Job drawing, mm, ordinate dimensions from the low corner. One solid piece. A direction names the side the tool comes from. Give positions to 0.01 mm unless a question says otherwise; leave off trailing zeros. Loops run counter-clockwise (first coordinate to the right, second up) from the corner with the lowest first, then second, coordinate; pieces in that order, holes last. Notation, with made-up numbers: M 4,-19 L 36,-19 A20 cw 36,13 Z; hole C 79.5,-10 d6. An arc over 180 degrees is marked long. Answer in a Markdown table with one row per item.
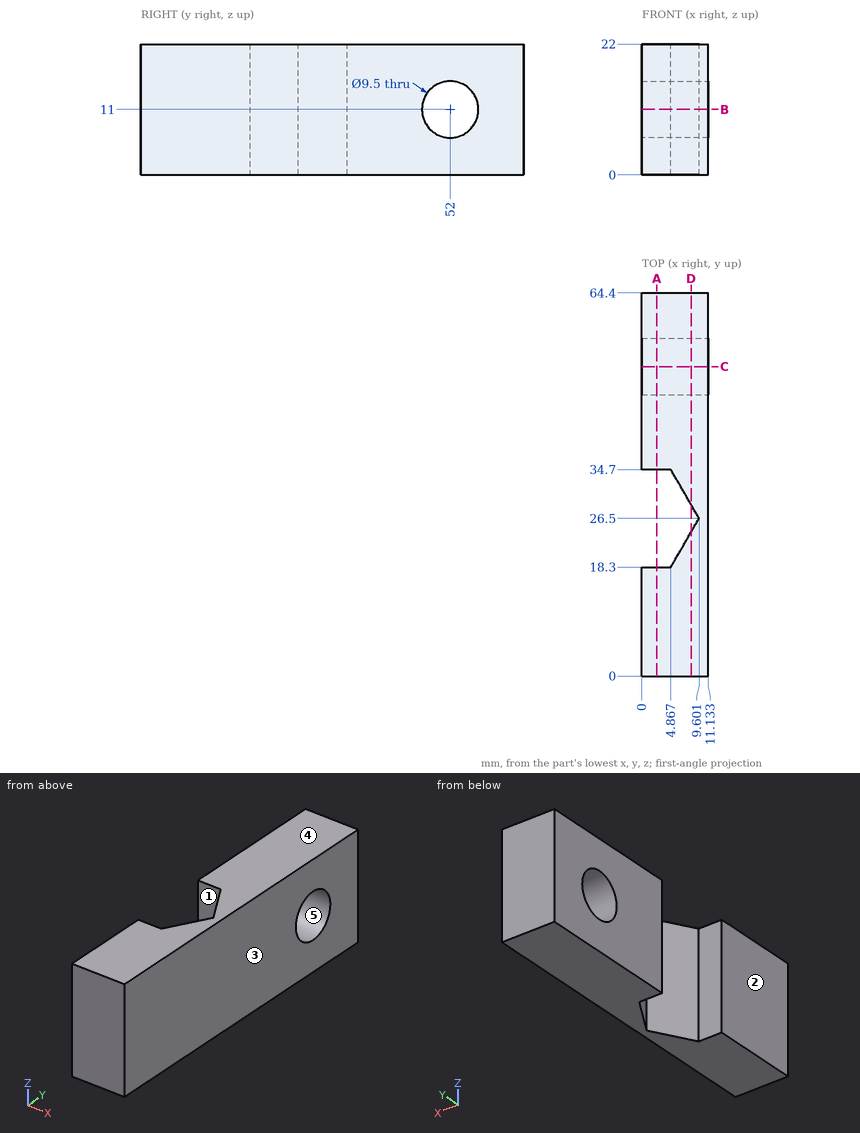
(1) Saw through at B-B (z = 11). Write the cut outline in (x, y).
Recorded:
| item | result |
|---|---|
| outline | M 0,0 L 11.13,0 L 11.13,47.25 L 0,47.25 L 0,34.7 L 4.87,34.7 L 9.6,26.5 L 4.87,18.3 L 0,18.3 Z; M 0,56.75 L 11.13,56.75 L 11.13,64.4 L 0,64.4 Z |
(2) Saw through at D-D (x = 8.25). Write the cut outline in (y, z).
Recorded:
| item | result |
|---|---|
| outline | M 0,0 L 24.16,0 L 24.16,22 L 0,22 Z; M 28.84,0 L 64.4,0 L 64.4,22 L 28.84,22 Z; hole C 52,11 d9.5 |
(3) Saw through at A-A (x = 2.5). Write the cut outline in (y, z), plus the area to 3 significant figures.
Recorded:
| item | result |
|---|---|
| outline | M 0,0 L 18.3,0 L 18.3,22 L 0,22 Z; M 34.7,0 L 64.4,0 L 64.4,22 L 34.7,22 Z; hole C 52,11 d9.5 |
| area | 985 mm^2 |
(4) Drill centre lines: line 1 along Y through (x, z) = (3, 11); line 2 along Y through (x, z) = (2.5, 4.25); line 3 along Y through (x, z) = (3.5, 9.5). Where is each one in solid material? Low to high.
Recorded:
| item | result |
|---|---|
| line 1 | y = 0 to 18.3, 34.7 to 47.25, 56.75 to 64.4 |
| line 2 | y = 0 to 18.3, 34.7 to 64.4 |
| line 3 | y = 0 to 18.3, 34.7 to 47.49, 56.51 to 64.4 |
(5) Which spindle directions (+Z, -Z, +X, -X, +Y, -Y) get a long thin tool onto all of the face, cutting with end or side? Do the marked faces 1 and 2. Say none if no direction does.
Recorded:
| item | result |
|---|---|
| face 1 | +Z, -Z, -X |
| face 2 | +Z, -Z, -X, +Y, -Y |
(6) Pull direction Z, two halves, no side cores. Call the marked faces 3, 4 and 5: +Z half, -Z half, draft (parallel to the pull), parting line (faces both ways), or undercut.
Recorded:
| item | result |
|---|---|
| face 3 | draft |
| face 4 | +Z half |
| face 5 | undercut |
(7) Pin check, flat tip, straight feed: pin 1 Ø1 at (y, z) = (24, 16) entering from -X. Stop position of the tip, or through.
Recorded:
| item | result |
|---|---|
| pin 1 | stops at x = 7.87 |
(8) Saw through at C-C (y = 52). Write the cut outline in (x, z), plus the area to 3 significant figures.
Recorded:
| item | result |
|---|---|
| outline | M 0,0 L 11.13,0 L 11.13,6.25 L 0,6.25 Z; M 0,15.75 L 11.13,15.75 L 11.13,22 L 0,22 Z |
| area | 139 mm^2 |
